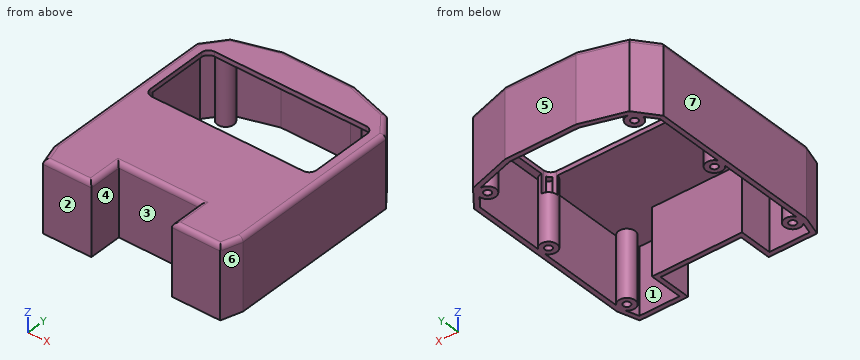
```python
from build123d import *

# Parameters (mm, degrees)
EXTRUDE_1_DEPTH     = 30
FILLET_4_R          = 2
SKETCH_2_R          = 1.5
CUT_EXTRUDE_1_DEPTH = 28
SHELL_3_DEPTH       = 28
CUT_EXTRUDE_2_DEPTH = 10


# Read off the part's stored shape, not the designer's step: 抽壳3
with BuildPart() as part:
    # 草图1 → 凸台-拉伸1 (new body)
    with BuildSketch(Plane.XY):
        Polygon((-84.402777778, 44), (-87, 52.5), (-87, 125.5), (-80, 134.5), (-62, 140), (-32, 140), (-14, 134.5), (-7, 125.5), (-7, 52.5), (-9.597222222, 44), (-30, 44), (-30, 58), (-64, 58), (-64, 44), align=None)
    extrude(amount=EXTRUDE_1_DEPTH)

    # 圆角4
    fillet_4_edges = [part.edges().sort_by_distance(p)[0] for p in [
        (-47, 58, 30),
        (-30, 51, 30),
        (-19.798611111, 44, 30),
        (-8.298611111, 48.25, 30),
        (-7, 89, 30),
        (-10.5, 130, 30),
        (-23, 137.25, 30),
        (-47, 140, 30),
        (-71, 137.25, 30),
        (-83.5, 130, 30),
        (-74.201388889, 44, 30),
        (-87, 89, 30),
        (-85.701388889, 48.25, 30),
        (-64, 51, 30),
    ]]
    fillet(fillet_4_edges, radius=FILLET_4_R)

    # 草图2 → 切除-拉伸1 (cut)
    with BuildSketch(Plane(origin=(0, 0, 0), x_dir=(-1, 0, 0), z_dir=(0, 0, -1))):
        with Locations((82, 53.5)):
            Circle(SKETCH_2_R)
        with Locations((12, 53.5)):
            Circle(SKETCH_2_R)
        with Locations((12, 93.5)):
            Circle(SKETCH_2_R)
        with Locations((82, 93.5)):
            Circle(SKETCH_2_R)
        with Locations((78, 129.5)):
            Circle(SKETCH_2_R)
        with Locations((16, 129.5)):
            Circle(SKETCH_2_R)
    extrude(amount=-CUT_EXTRUDE_1_DEPTH, mode=Mode.SUBTRACT)

    # 抽壳3 outline → 抽壳3 (cut)
    with BuildSketch(Plane.XY):
        with BuildLine():
            Line((-9, 55.302775638), (-9, 91.697224362))
            ThreePointArc((-9, 91.697224362), (-15.5, 93.5), (-9, 95.302775638))
            Line((-9, 95.302775638), (-9, 124.8137845))
            Line((-9, 124.8137845), (-12.504644228, 129.31975565))
            ThreePointArc((-12.504644228, 129.31975565), (-18.560753547, 127.114095293), (-15.933003152, 132.999358716))
            Line((-15.933003152, 132.999358716), (-32.298738264, 138))
            Line((-32.298738264, 138), (-61.701261736, 138))
            Line((-61.701261736, 138), (-78.066996848, 132.999358716))
            ThreePointArc((-78.066996848, 132.999358716), (-75.439246453, 127.114095293), (-81.495355772, 129.31975565))
            Line((-81.495355772, 129.31975565), (-85, 124.8137845))
            Line((-85, 124.8137845), (-85, 95.302775638))
            ThreePointArc((-85, 95.302775638), (-78.5, 93.5), (-85, 91.697224362))
            Line((-85, 91.697224362), (-85, 55.302775638))
            ThreePointArc((-85, 55.302775638), (-78.528186006, 53.943291769), (-84.450768591, 51.001253651))
            Line((-84.450768591, 51.001253651), (-82.922607753, 46))
            Line((-82.922607753, 46), (-66, 46))
            Line((-66, 46), (-66, 60))
            Line((-66, 60), (-28, 60))
            Line((-28, 60), (-28, 46))
            Line((-28, 46), (-11.077392247, 46))
            Line((-11.077392247, 46), (-9.549231409, 51.001253651))
            ThreePointArc((-9.549231409, 51.001253651), (-15.471813994, 53.943291769), (-9, 55.302775638))
        make_face()
    extrude(amount=SHELL_3_DEPTH, mode=Mode.SUBTRACT)

    # 草图3 → 切除-拉伸2 (cut)
    with BuildSketch(Plane.XY.offset(30)):
        with BuildLine():
            Line((-79, 125), (-15, 125))
            ThreePointArc((-15, 125), (-12.878679656, 124.121320344), (-12, 122))
            Line((-12, 122), (-12, 96))
            ThreePointArc((-12, 96), (-12.878679656, 93.878679656), (-15, 93))
            Line((-15, 93), (-79, 93))
            ThreePointArc((-79, 93), (-81.121320344, 93.878679656), (-82, 96))
            Line((-82, 96), (-82, 122))
            ThreePointArc((-82, 122), (-81.121320344, 124.121320344), (-79, 125))
        make_face()
    extrude(amount=-CUT_EXTRUDE_2_DEPTH, mode=Mode.SUBTRACT)


solid = part.part
```
Geometry check sheet. Reference: the model listing, model coordinates, mm. Face numbers are marked on the shaded views. A direction names the side the tool comes from. Coordinates: 2 decimals unless noted, no trailing zeros. Write each loop counter-clockwise with the first axis right and the second up, starting at its lowest first coordinate (ties: lowest second). Pieces come first, ordered by that corner, then holes. Notation, with made-up numbers: M -37.75,44.5 L -29.75,44.5 A32 cw -29.75,76.5 Z; hole C 81.25,11.25 d9. An arc over 180 degrees is marked long. Use one line per item in the form item = value. Start each with the question number.
1) Section check A-A on x = -55.5. Enter the section's corners in (y, z), and give its area (3 significant figures).
2) Release check for a two-part mould opening along X. For the marked faces 4, 5, 6 and 7 record: pulls with the +X half, pulls with the -X half, needs draft (parallel to the pull), parting line crosses it, or undercut.
3) Set-up check for the marked faces 1, 2 and 3: record each of +Z, -Z, +X, -X, +Y, -Y from which the full face is reachable in a straight line by a thin tool's end or side.
4) Section check C-C on z = 3.5. State how many separate pieces and enclosed holes the cut face has, and give its area (3 significant figures).
5) Thickness scan on probe 1 along Y at (x, z) = (-59, 12); probe 2 along X at (y, z) = (67, 5.25); probe 3 along X at (y, z) = (56.5, 18.5). Record the ranges inside material, lowest first. Write a range as from..to.
6) Section check B-B on y = 110.5. Enter the section's corners in (x, z).
7) Go/stop test with flat-tipped pins: pin 1 Ø0.9 at (x, y) = (-82.5, 53) entering from -Z; pin 2 Ø13.5 at (x, z) = (-24, 16) entering from +Y; pin 3 Ø3 at (x, z) = (-74, 8.5) entering from +Y. Record where each tip stops, or that it passes through.
Responses:
q1.outline = M 58,0 L 60,0 L 60,28 L 93,28 L 93,30 L 60,30 A2 ccw 58,28 Z; M 125,28 L 138,28 L 138,0 L 140,0 L 140,28 A2 ccw 138,30 L 125,30 Z
q1.area = 210 mm2
q2.face_4 = undercut
q2.face_5 = needs draft
q2.face_6 = pulls with the +X half
q2.face_7 = pulls with the -X half
q3.face_1 = -Z
q3.face_2 = +Z, -Z, +X, -X, -Y
q3.face_3 = +Z, -Z, -Y
q4.separate_pieces = 1
q4.enclosed_holes = 7
q4.area = 878 mm2
q5.probe_1 = 58..60, 138..140
q5.probe_2 = -87..-85, -9..-7
q5.probe_3 = -87..-85, -83.8..-80.2, -66..-64, -30..-28, -13.8..-10.2, -9..-7
q6.outline = M -87,0 L -85,0 L -85,28 L -82,28 L -82,30 L -85,30 A2 ccw -87,28 Z; M -12,28 L -9,28 L -9,0 L -7,0 L -7,28 A2 ccw -9,30 L -12,30 Z
q7.pin_1 = 28
q7.pin_2 = 139.62
q7.pin_3 = 136.79
